Design review of the part built by this model. Coordinates are the model's own, in mm. A direction names the side the tool comes from. Coordinates: 2 decimals unless noted, no trailing zeros. Write each loop counter-clockwise with the first axis right and the second up, starting at its lowest first coordinate (ties: lowest second). Pieces come first, ordered by that corner, then holes. Notation, with made-up numbers: (-20, 32) - (37, 32) arc R21 ccw to (37, 47) - close; hole circle Ø9 at (25, 53). An arc over 180 degrees is marked (long way). Answer as a JSON object with one key per item and string values.
```python
from build123d import *

# Parameters (mm, degrees)
SALIENTE_EXTRUIR1_DEPTH      = 118.5
SALIENTE_EXTRUIR1_DEPTH_BACK = 118.5
CROQUIS1_R                   = 16
CROQUIS1_R_2                 = 3.65


with BuildPart() as part:
    # Croquis1 → Saliente-Extruir1 (new, two sides: drawn at the far end of the back side and taken through both)
    with BuildSketch(Plane(origin=(0, 0, 0), x_dir=(1, 0, 0), z_dir=(0, 1, 0)).offset(-SALIENTE_EXTRUIR1_DEPTH_BACK)):
        with BuildLine():
            Line((22.519467165, 2.803307997), (22.519467165, 5.703307997))
            Line((22.519467165, 5.703307997), (22.360287832, 6.103307997))
            Line((22.360287832, 6.103307997), (21.060287832, 5.585975165))
            Line((21.060287832, 5.585975165), (21.282135886, 5.028495622))
            Line((21.282135886, 5.028495622), (17.782135886, 3.635676459))
            ThreePointArc((17.782135886, 3.635676459), (16.78664035, 6.901536477), (15.197137425, 9.923180644))
            Line((15.197137425, 9.923180644), (18.634927939, 11.291243646))
            Line((18.634927939, 11.291243646), (18.856775994, 10.733764103))
            Line((18.856775994, 10.733764103), (20.064648337, 11.214434887))
            Line((20.064648337, 11.214434887), (19.510028201, 12.608133745))
            ThreePointArc((19.510028201, 12.608133745), (20.45236818, 13.820216674), (20.984473879, 15.260360134))
            Line((20.984473879, 15.260360134), (22.284473879, 15.260360134))
            Line((22.284473879, 15.260360134), (22.284473879, 17.260360134))
            Line((22.284473879, 17.260360134), (20.984473879, 17.260360134))
            ThreePointArc((20.984473879, 17.260360134), (17.580307493, 21.047671527), (12.616069545, 19.912586524))
            Line((12.616069545, 19.912586524), (8.656271571, 15.952788549))
            ThreePointArc((8.656271571, 15.952788549), (0, 18.15), (-8.656271571, 15.952788549))
            Line((-8.656271571, 15.952788549), (-12.616069545, 19.912586524))
            ThreePointArc((-12.616069545, 19.912586524), (-17.580307493, 21.047671527), (-20.984473879, 17.260360134))
            Line((-20.984473879, 17.260360134), (-22.284473879, 17.260360134))
            Line((-22.284473879, 17.260360134), (-22.284473879, 15.260360134))
            Line((-22.284473879, 15.260360134), (-20.984473879, 15.260360134))
            ThreePointArc((-20.984473879, 15.260360134), (-20.45236818, 13.820216674), (-19.510028201, 12.608133745))
            Line((-19.510028201, 12.608133745), (-20.064648337, 11.214434887))
            Line((-20.064648337, 11.214434887), (-18.856775994, 10.733764103))
            Line((-18.856775994, 10.733764103), (-18.634927939, 11.291243646))
            Line((-18.634927939, 11.291243646), (-15.197137425, 9.923180644))
            ThreePointArc((-15.197137425, 9.923180644), (-16.78664035, 6.901536477), (-17.782135886, 3.635676459))
            Line((-17.782135886, 3.635676459), (-21.282135886, 5.028495622))
            Line((-21.282135886, 5.028495622), (-21.060287832, 5.585975165))
            Line((-21.060287832, 5.585975165), (-22.360287832, 6.103307997))
            Line((-22.360287832, 6.103307997), (-22.519467165, 5.703307997))
            Line((-22.519467165, 5.703307997), (-22.519467165, 2.803307997))
            Line((-22.519467165, 2.803307997), (-18.119467165, 1.052335335))
            ThreePointArc((-18.119467165, 1.052335335), (-18.15, 0), (-18.119467165, -1.052335335))
            Line((-18.119467165, -1.052335335), (-22.519467165, -2.803307997))
            Line((-22.519467165, -2.803307997), (-22.519467165, -5.703307997))
            Line((-22.519467165, -5.703307997), (-22.360287832, -6.103307997))
            Line((-22.360287832, -6.103307997), (-21.060287832, -5.585975165))
            Line((-21.060287832, -5.585975165), (-21.282135886, -5.028495622))
            Line((-21.282135886, -5.028495622), (-17.782135886, -3.635676459))
            ThreePointArc((-17.782135886, -3.635676459), (-16.78664035, -6.901536477), (-15.197137425, -9.923180644))
            Line((-15.197137425, -9.923180644), (-18.634927939, -11.291243646))
            Line((-18.634927939, -11.291243646), (-18.856775994, -10.733764103))
            Line((-18.856775994, -10.733764103), (-20.064648337, -11.214434887))
            Line((-20.064648337, -11.214434887), (-19.510028201, -12.608133745))
            ThreePointArc((-19.510028201, -12.608133745), (-20.45236818, -13.820216674), (-20.984473879, -15.260360134))
            Line((-20.984473879, -15.260360134), (-22.284473879, -15.260360134))
            Line((-22.284473879, -15.260360134), (-22.284473879, -17.260360134))
            Line((-22.284473879, -17.260360134), (-20.984473879, -17.260360134))
            ThreePointArc((-20.984473879, -17.260360134), (-18.321863215, -20.745689761), (-13.936329401, -20.809809373))
            Line((-13.936329401, -20.809809373), (-10.255447151, -20.809809373))
            Line((-10.255447151, -20.809809373), (-10.255447151, -19.109809373))
            ThreePointArc((-10.255447151, -19.109809373), (-8.705447151, -16.109151592), (-7.155447151, -19.109809373))
            Line((-7.155447151, -19.109809373), (-7.155447151, -20.809809373))
            Line((-7.155447151, -20.809809373), (-5.555447151, -20.809809373))
            Line((-5.555447151, -20.809809373), (-4.41427266, -17.605019082))
            ThreePointArc((-4.41427266, -17.605019082), (0, -18.15), (4.41427266, -17.605019082))
            Line((4.41427266, -17.605019082), (5.555447151, -20.809809373))
            Line((5.555447151, -20.809809373), (7.155447151, -20.809809373))
            Line((7.155447151, -20.809809373), (7.155447151, -19.109809373))
            ThreePointArc((7.155447151, -19.109809373), (8.705447151, -16.109151592), (10.255447151, -19.109809373))
            Line((10.255447151, -19.109809373), (10.255447151, -20.809809373))
            Line((10.255447151, -20.809809373), (13.936329401, -20.809809373))
            ThreePointArc((13.936329401, -20.809809373), (18.321863215, -20.745689761), (20.984473879, -17.260360134))
            Line((20.984473879, -17.260360134), (22.284473879, -17.260360134))
            Line((22.284473879, -17.260360134), (22.284473879, -15.260360134))
            Line((22.284473879, -15.260360134), (20.984473879, -15.260360134))
            ThreePointArc((20.984473879, -15.260360134), (20.45236818, -13.820216674), (19.510028201, -12.608133745))
            Line((19.510028201, -12.608133745), (20.064648337, -11.214434887))
            Line((20.064648337, -11.214434887), (18.856775994, -10.733764103))
            Line((18.856775994, -10.733764103), (18.634927939, -11.291243646))
            Line((18.634927939, -11.291243646), (15.197137425, -9.923180644))
            ThreePointArc((15.197137425, -9.923180644), (16.78664035, -6.901536477), (17.782135886, -3.635676459))
            Line((17.782135886, -3.635676459), (21.282135886, -5.028495622))
            Line((21.282135886, -5.028495622), (21.060287832, -5.585975165))
            Line((21.060287832, -5.585975165), (22.360287832, -6.103307997))
            Line((22.360287832, -6.103307997), (22.519467165, -5.703307997))
            Line((22.519467165, -5.703307997), (22.519467165, -2.803307997))
            Line((22.519467165, -2.803307997), (18.119467165, -1.052335335))
            ThreePointArc((18.119467165, -1.052335335), (18.15, 0), (18.119467165, 1.052335335))
            Line((18.119467165, 1.052335335), (22.519467165, 2.803307997))
        make_face()
        with Locations(Location((0, 0, 0), (0, 0, 270))):
            Circle(CROQUIS1_R, mode=Mode.SUBTRACT)
        with Locations(Location((16.063048873, 16.260360134, 0), (0, 0, 270))):
            Circle(CROQUIS1_R_2, mode=Mode.SUBTRACT)
        with Locations(Location((-16.063048873, 16.260360134, 0), (0, 0, 90))):
            Circle(CROQUIS1_R_2, mode=Mode.SUBTRACT)
        with Locations(Location((-16.063048873, -16.260360134, 0), (0, 0, 270))):
            Circle(CROQUIS1_R_2, mode=Mode.SUBTRACT)
        with Locations(Location((16.063048873, -16.260360134, 0), (0, 0, 90))):
            Circle(CROQUIS1_R_2, mode=Mode.SUBTRACT)
    extrude(amount=SALIENTE_EXTRUIR1_DEPTH + SALIENTE_EXTRUIR1_DEPTH_BACK)


solid = part.part
```
(1) Tool access review of faces 1 (the face through (-20.289, -1.659, 1.916)), 2 (the face through (13.842, -1.659, -19.157)), 3 (the face through (20.35, -1.66, 1.94)), 4 (the face through (10.664, -1.659, -17.96)): name each direction out of +Z, -Z, +X, -X, +Y, -Y from which nothing blocks a thin tool from reaching the whole face with its end or side.
Solved:
{"face 1": "-X, +Y, -Y", "face 2": "+Y, -Y", "face 3": "+X, +Y, -Y", "face 4": "-Z, +Y, -Y"}
(2) The part is to be moulded in two halves that separate along X. For faces 5 (the face through (-20.35, -1.66, -1.94)), 6 (the face through (-8.76, -1.66, 16.11)), 7 (the face through (-3, 118.5, 16)), say which applies: pulls with the +X half, pulls with the -X half, needs draft (parallel to the pull), parting line crosses it, or undercut.
Solved:
{"face 5": "pulls with the -X half", "face 6": "undercut", "face 7": "needs draft"}
(3) Take a section at B-B, the plane y = 41. Give the number of separate pieces and of enclosed holes in the cut face, and give its area (3 significant figures).
Solved:
{"separate pieces": "1", "enclosed holes": "5", "area": "507 mm^2"}
(4) For pin 1 (3 mm diameter, centred on x = 1.5, y = 70, fed in from -Z); pin 2 (1 mm diameter, centred on x = -8.5, y = 35, fed in from +Z); pin 3 (1.1 mm diameter, centred on x = 12.5, y = 5.5, fed in from +Z); pin 4 (2.5 mm diameter, centred on x = 8.71, z = 18.01, fed in from -Y), all flat-tipped, find the tip position at first contact; note any pin that passes through.
Solved:
{"pin 1": "stops at z = -18.15", "pin 2": "stops at z = 16.24", "pin 3": "stops at z = 20.81", "pin 4": "passes through"}
(5) To check wall thickness, follow line 1 (Z direction, x = -14, y = 82); line 2 (Z direction, x = -18, y = 4); line 3 (X direction, y = 29.5, z = -14.5). State the ranges of each line that lie inside material, in increasing order. Write a range as from..to.
Solved:
{"line 1": "z = -20.84..-19.27, -13.25..-7.75, 7.75..13.25, 19.27..20.84", "line 2": "z = -20.89..-19.35, -13.17..-11.04, -3.72..3.72, 11.04..13.17, 19.35..20.89", "line 3": "x = -20.77..-19.26, -12.87..-6.76, 6.76..12.87, 19.26..20.77"}
(6) Take a section at A-A, the plane x = 0. Write out the cut boundary in (y, z), and give its area (3 significant figures).
Solved:
{"outline": "(-118.5, -18.15) - (118.5, -18.15) - (118.5, -16) - (-118.5, -16) - close; (-118.5, 16) - (118.5, 16) - (118.5, 18.15) - (-118.5, 18.15) - close", "area": "1,020 mm^2"}
